Check sheet for the modelled part. Datum: model origin and axes. Units: mm. A direction names the side the tool comes from. Give positions to 0.01 mm unless a question says otherwise; leave off trailing zeros. Write each loop counter-clockwise with the first axis right and the second up, starting at its lowest first coordinate (ties: lowest second). Pieces come first, ordered by that corner, then holes. Notation, with made-up numbers: M -5.5,48 L 20.5,48 A15 cw 20.5,59 Z; hole C 12.5,77.5 d9. An arc over 180 degrees is marked long. Use CSV: the item, a comma, the result in double quotes. Start each with the question number.
1. Scan lines: line 1 (Z direction, x = -4.75, y = -6); line 2 (X direction, y = 2, z = 71.5); line 3 (X direction, y = -1.25, z = 59). Record each from-to range of solid material in increasing order.
2. Depth check by flat-ended pin: P1, Ø3, axis at y = -2.5, z = 57, coming from the -X side; P2, Ø6, axis at x = -4.5, y = 0.5, coming from the +Z side; P3, Ø2, axis at x = 5, z = 76.5, coming from the -Y side. Enter the tip coordinate at first touch or a pass-through.
3. Cross-section at B-B, the plane x = -6. Enter the section's corners in (y, z).
4. Cross-section at A-A, the plane z = 26. Enter the section's corners in (x, y).
5. Access from +Z, -Z, +X, -X, +Y, -Y to the whole of each face (thin tool, end or side, straight path). Record for faces 1 (the face through (0, 0, 0)), 2 (the face through (-1.08, -4.88, 51.33)).
6. Cross-section at C-C, the plane x = 6.5. Enter the section's corners in (y, z), and give its area (3 significant figures).
from build123d import *

# Parameters (mm, degrees)
F0_R     = 8.5
F1_DEPTH = 4
F2_R     = 5
F3_DEPTH = 100


with BuildPart() as f1:
    # F0 (on Top) → F1 (new body)
    with BuildSketch(Plane.XY):
        Circle(F0_R)
    extrude(amount=F1_DEPTH)

    # F2 (on Top) → F3 (join)
    with BuildSketch(Plane.XY):
        Circle(F2_R)
    extrude(amount=F3_DEPTH)

    # F4 (on Right) → F5 (revolve)
    with BuildSketch(Plane.YZ):
        with BuildLine():
            Line((3, 102), (0, 102))
            Line((0, 102), (0, 100))
            Line((0, 100), (5, 100))
            ThreePointArc((5, 100), (3.585786, 100.585786), (3, 102))
        make_face()
    revolve(axis=Axis((0, 0, 101), (0, 0, -1)))

    # F6 (on Right) → F7 (revolve)
    with BuildSketch(Plane.YZ):
        with BuildLine():
            Line((0, 105), (0, 102))
            Line((0, 102), (3, 102))
            ThreePointArc((3, 102), (2.12132, 104.12132), (0, 105))
        make_face()
    revolve(axis=Axis((0, 0, 103.5), (0, 0, 1)))


solid = f1.part
Worked answers:
1,line 1,"z = 0 to 4"
1,line 2,"x = -4.58 to 4.58"
1,line 3,"x = -4.84 to 4.84"
2,P1,"stops at x = -4.9"
2,P2,"stops at z = 104.58"
2,P3,"stops at y = -3"
3,outline,"M -6.02,0 L 6.02,0 L 6.02,4 L -6.02,4 Z"
4,outline,"C 0,0 d10"
5,face 1,"-Z, +X, -X, +Y, -Y"
5,face 2,"+Z"
6,outline,"M -5.48,0 L 5.48,0 L 5.48,4 L -5.48,4 Z"
6,area,"43.8 mm^2"
